from build123d import *

# Parameters (mm, degrees)
SKETCH1_R           = 10
BOSS_EXTRUDE1_DEPTH = 12.2
SKETCH4_R           = 2.5
BOSS_EXTRUDE3_DEPTH = 0.5
SKETCH5_R           = 1
BOSS_EXTRUDE4_DEPTH = 3.32
FILLET1_R           = 6
SKETCH2_R           = 3
BOSS_EXTRUDE2_DEPTH = 4
SKETCH6_R           = 2.25
CUT_EXTRUDE1_DEPTH  = 2.55


with BuildPart() as part:
    # Sketch1 → Boss-Extrude1 (new body)
    with BuildSketch(Plane.XY):
        Circle(SKETCH1_R)
    extrude(amount=BOSS_EXTRUDE1_DEPTH)

    # Sketch4 → Boss-Extrude3 (add)
    with BuildSketch(Plane.XY.offset(12.2)):
        Circle(SKETCH4_R)
    extrude(amount=BOSS_EXTRUDE3_DEPTH)

    # Sketch5 → Boss-Extrude4 (add)
    with BuildSketch(Plane.XY.offset(12.2)):
        with Locations(Location((0, 0, 0), (0, 0, 180))):
            Circle(SKETCH5_R)
    extrude(amount=BOSS_EXTRUDE4_DEPTH)

    # Fillet1
    fillet1_edges = [part.edges().sort_by_distance(p)[0] for p in [
        (-10, 0, 0),
        (-10, 0, 12.2),
    ]]
    fillet(fillet1_edges, radius=FILLET1_R)

    # Sketch2 → Boss-Extrude2 (add)
    with BuildSketch(Plane(origin=(0, 0, 0), x_dir=(-1, 0, 0), z_dir=(0, 0, -1))):
        with Locations(Location((0, 0, 0), (0, 0, 180))):
            Circle(SKETCH2_R)
    extrude(amount=BOSS_EXTRUDE2_DEPTH)

    # Sketch6 → Cut-Extrude1 (cut)
    with BuildSketch(Plane(origin=(0, 0, -4), x_dir=(-1, 0, 0), z_dir=(0, 0, -1))):
        Circle(SKETCH6_R)
    extrude(amount=-CUT_EXTRUDE1_DEPTH, mode=Mode.SUBTRACT)

    # Sketch7 → Cut-Revolve1 (revolve, cut)
    with BuildSketch(Plane(origin=(0, 0, 0), x_dir=(0, 0, -1), z_dir=(1, 0, 0)), mode=Mode.PRIVATE) as cut_revolve1_sk:
        with BuildLine():
            Line((-7.887262955, 10.599100827), (-4.29107992, 10.599100827))
            Line((-4.29107992, 10.599100827), (-4.29107992, 9.471207056))
            ThreePointArc((-4.29107992, 9.471207056), (-6.089171437, 9.757850623), (-7.887262955, 9.471207056))
            Line((-7.887262955, 9.471207056), (-7.887262955, 10.599100827))
        make_face()
    revolve(cut_revolve1_sk.sketch.rotate(Axis((0, 0, 15.193399994), (0, 0, -1)), 90), axis=Axis((0, 0, 15.193399994), (0, 0, -1)), mode=Mode.SUBTRACT)


solid = part.part
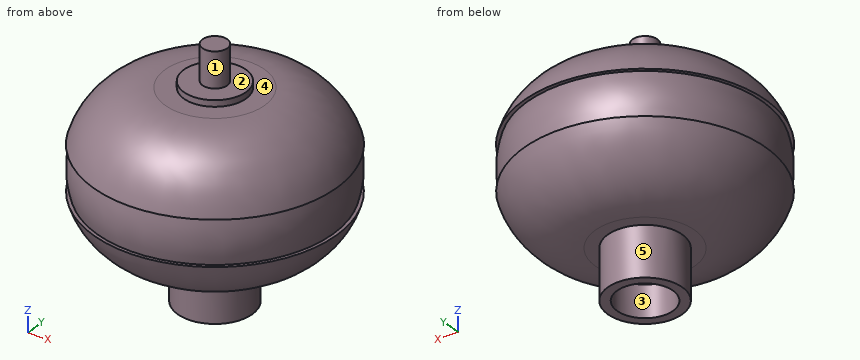
Geometry: final body of the model. Coordinates: model frame, mm. Face numbers are marked on the shaded views. A direction names the side the tool comes from. Round coordinates to 2 decimals unless told otherwise and drop trailing zeros. Loops run counter-clockwise (first coordinate to the right, second up) from the corner with the lowest first, then second, coordinate; pieces in that order, holes last. Notation, with made-up numbers: M 87.5,79.25 L 134.5,79.25 A20 ccw 134.5,99.25 Z; hole C 35,32 d11. An arc over 180 degrees is marked long. One line per question, with ' | ' between items.
(1) Contact query for flat-ended pins moving along their axis: P1, Ø5, axis at y = 4.5, z = 12.5, coming from the -X side; P2, Ø6, axis at y = -3.5, z = 10.5, coming from the +X side; P3, Ø1.3, axis at x = 0, y = 0.5, coming from the -Z side. Output: stop coordinate, or through.
Check result:
P1: stops at x = -7.71 | P2: stops at x = 9.55 | P3: stops at z = -1.45
(2) Material intervals for line 1 along Y through (x, z) = (0, -2.4); line 2 along Z through (x, y) = (-1.75, 3); line 3 along Z through (x, y) = (1.25, 0), sorted ascending. Write a range as from..to.
Check result:
line 1: y = -3..-2.25, 2.25..3 | line 2: z = 0..12.2 | line 3: z = -1.45..12.7
(3) Access query for the marked faces 4 and 5. Directions: +Z, -Z, +X, -X, +Y, -Y. A direction counts if a zero-diameter tool reaches every point of the face in a straight line with its end or side. Return the directions, or none.
Check result:
face 4: +Z | face 5: -Z
(4) Pull-direction query (X, two-part tool) for the marked faces 1, 2 and 3; classes: +X half, -X half, draft (parallel to the pull), parting line (faces both ways), or undercut.
Check result:
face 1: parting line | face 2: draft | face 3: undercut
(5) Cut plane A-A on z = 13.25. Return the cut outline in (x, y).
Check result:
outline: C 0,0 d2
